```python
from build123d import *

# Parameters (mm, degrees)
F0_W     = 69.85
F0_H     = 76.2
F0_R     = 2.5
F0_R_2   = 19.05
F1_DEPTH = 3.175
F0_W_2   = 3.175
F2_DEPTH = 127
F3_R     = 1.778
F3_R_2   = 4.7625
F4_DEPTH = 76.201
F5_R     = 25.4
F6_R     = 25.4
F7_R     = 25.4
F8_R     = 25.4


with BuildPart() as f1:
    # F0 (on Front) → F1 (new body)
    with BuildSketch(Plane.XZ):
        Rectangle(F0_W, F0_H)
        with Locations((-23.5, -23.5)):
            Circle(F0_R, mode=Mode.SUBTRACT)
        with Locations((23.5, -23.5)):
            Circle(F0_R, mode=Mode.SUBTRACT)
        with Locations((-23.5, 23.5)):
            Circle(F0_R, mode=Mode.SUBTRACT)
        Circle(F0_R_2, mode=Mode.SUBTRACT)
        with Locations((23.5, 23.5)):
            Circle(F0_R, mode=Mode.SUBTRACT)
    extrude(amount=F1_DEPTH)

    # F0 (on Front) → F2 (join)
    with BuildSketch(Plane.XZ):
        with Locations((-36.5125, 0)):
            Rectangle(F0_W_2, F0_H)
        with Locations((36.5125, 0)):
            Rectangle(F0_W_2, F0_H)
    extrude(amount=F2_DEPTH)

    # F3 (on face) → F4 (cut, through all)
    with BuildSketch(Plane.YZ.offset(38.1)):
        with Locations((-120.65, 6.9088)):
            Circle(F3_R)
        with Locations((-106.8324, 6.9088)):
            Circle(F3_R)
        with Locations((-106.8324, -6.9088)):
            Circle(F3_R)
        with Locations((-120.65, -6.9088)):
            Circle(F3_R)
        with Locations((-113.7412, 0)):
            Circle(F3_R_2)
    extrude(amount=-F4_DEPTH, mode=Mode.SUBTRACT)

    # F5
    f5_edges = [f1.edges().sort_by_distance(p)[0] for p in [
        (36.5125, -127, 38.1),
    ]]
    fillet(f5_edges, radius=F5_R)

    # F6
    f6_edges = [f1.edges().sort_by_distance(p)[0] for p in [
        (-36.5125, -127, 38.1),
    ]]
    fillet(f6_edges, radius=F6_R)

    # F7
    f7_edges = [f1.edges().sort_by_distance(p)[0] for p in [
        (-36.5125, -127, -38.1),
    ]]
    fillet(f7_edges, radius=F7_R)

    # F8
    f8_edges = [f1.edges().sort_by_distance(p)[0] for p in [
        (36.5125, -127, -38.1),
    ]]
    fillet(f8_edges, radius=F8_R)


solid = f1.part
```
Check sheet for the modelled part. Datum: model origin and axes. Units: mm. A direction names the side the tool comes from. Coordinates: 2 decimals unless noted, no trailing zeros. Write each loop counter-clockwise with the first axis right and the second up, starting at its lowest first coordinate (ties: lowest second). Pieces come first, ordered by that corner, then holes. Notation, with made-up numbers: (25, 38.25) -> (57, 38.25) arc R16 ccw to (57, 66.25) -> close; hole circle Ø8 at (2, 66). An arc over 180 degrees is marked (long way). Use a Markdown table: item, result.
1. Sectioned sample at C-C (z = 0). Enter the section's corners in (x, y) (3 decimals).
Reported:
| item | result |
|---|---|
| outline | (-38.1, -127) -> (-34.925, -127) -> (-34.925, -118.504) -> (-38.1, -118.504) -> close; (-38.1, -108.979) -> (-34.925, -108.979) -> (-34.925, -3.175) -> (-19.05, -3.175) -> (-19.05, 0) -> (-38.1, 0) -> close; (19.05, -3.175) -> (34.925, -3.175) -> (34.925, -108.979) -> (38.1, -108.979) -> (38.1, 0) -> (19.05, 0) -> close; (34.925, -127) -> (38.1, -127) -> (38.1, -118.504) -> (34.925, -118.504) -> close |
2. Scan lines: line 1 along X through (y, z) = (-85.5, -20) (3 decimals); line 2 along X through (y, z) = (-1, 23); line 3 along Z through (x, y) = (0, -2.25). Record each from-to range of solid material in increasing order.
Reported:
| item | result |
|---|---|
| line 1 | x = -38.1 to -34.925, 34.925 to 38.1 |
| line 2 | x = -38.1 to -25.95, -21.05 to 21.05, 25.95 to 38.1 |
| line 3 | z = -38.1 to -19.05, 19.05 to 38.1 |
3. Sectioned sample at B-B (x = -23.5). Enter the section's corners in (y, z) (3 decimals).
Reported:
| item | result |
|---|---|
| outline | (-3.175, -38.1) -> (0, -38.1) -> (0, -26) -> (-3.175, -26) -> close; (-3.175, -21) -> (0, -21) -> (0, 21) -> (-3.175, 21) -> close; (-3.175, 26) -> (0, 26) -> (0, 38.1) -> (-3.175, 38.1) -> close |
4. Sectioned sample at D-D (x = 0). Enter the section's corners in (y, z) (3 decimals), plus the area to 3 significant figures.
Reported:
| item | result |
|---|---|
| outline | (-3.175, -38.1) -> (0, -38.1) -> (0, -19.05) -> (-3.175, -19.05) -> close; (-3.175, 19.05) -> (0, 19.05) -> (0, 38.1) -> (-3.175, 38.1) -> close |
| area | 121 mm2 |
5. Sectioned sample at A-A (y = -90). Enter the section's corners in (x, z) (3 decimals).
Reported:
| item | result |
|---|---|
| outline | (-38.1, -38.1) -> (-34.925, -38.1) -> (-34.925, 38.1) -> (-38.1, 38.1) -> close; (34.925, -38.1) -> (38.1, -38.1) -> (38.1, 38.1) -> (34.925, 38.1) -> close |
6. Go/stop test with flat-tipped pins: pin 1 Ø3 at (y, z) = (-120.65, 6.91) entering from -X; pin 2 Ø6 at (x, z) = (15, -7.5) entering from +Y. Record where each tip stops, or that it passes through.
Reported:
| item | result |
|---|---|
| pin 1 | passes through |
| pin 2 | stops at y = 0 |
7. Release check for a two-part mould opening along Z. For faces 3 (the cylindrical face through (-36.49, -119.76, -30.46)), 4 (the cylindrical face through (36.535, -122.426, -6.831)), 5 (the flat face through (-38.1, -63, -1)) record: pulls with the +Z half, pulls with the -Z half, needs draft (parallel to the pull), parting line crosses it, or undercut.
Reported:
| item | result |
|---|---|
| face 3 | pulls with the -Z half |
| face 4 | undercut |
| face 5 | needs draft |
8. Tool access check on faces 1 (the flat face through (34.925, -64, -1)), 2 (the cylindrical face through (-36.49, -122.426, -6.831)). Record the directions out of +Z, -Z, +X, -X, +Y, -Y that give a thin tool (end or side, any length) a straight path to the whole face; none if there is none.
Reported:
| item | result |
|---|---|
| face 1 | +Z, -Z, -Y |
| face 2 | +X, -X |
